Model file for the job. Use its own axes, mm. Coordinates: 2 decimals unless noted, no trailing zeros. Loops run counter-clockwise (first coordinate to the right, second up) from the corner with the lowest first, then second, coordinate; pieces in that order, holes last. Notation, with made-up numbers: (64.5, 7.5) -> (113.5, 7.5) arc R33 ccw to (113.5, 38.5) -> close; hole circle Ø9 at (78.5, -25). An arc over 180 degrees is marked (long way). Use one line per item in the form item = value.
```python
from build123d import *

# Parameters (mm, degrees)
F0_W     = 80
F0_H     = 80
F1_DEPTH = 3
F2_D     = 5.2
F3_R     = 10


with BuildPart() as f1:
    # F0 (on Top) → F1 (new body)
    with BuildSketch(Plane.XY):
        Rectangle(F0_W, F0_H)
    extrude(amount=F1_DEPTH)

    # F2 (through all)
    with Locations(Plane(origin=(0, 0, 0), x_dir=(1, 0, 0), z_dir=(0, 0, -1))):
        with Locations((-30, 30), (-10, 30), (10, 30), (30, 30), (30, 10), (10, 10), (-10, 10), (-30, 10), (-30, -10), (-10, -10), (10, -10), (30, -10), (30, -30), (10, -30), (-10, -30), (-30, -30)):
            Hole(F2_D / 2)

    # F3
    f3_edges = [f1.edges().sort_by_distance(p)[0] for p in [
        (40, 40, 1.5),
        (-40, 40, 1.5),
        (-40, -40, 1.5),
        (40, -40, 1.5),
    ]]
    fillet(f3_edges, radius=F3_R)


solid = f1.part
```
Q1. Band-saw the part on D-D, the plane x = -35. Write the cut outline in (y, z), and give its area (3 significant figures).
Result:
outline = (-38.66, 0) -> (38.66, 0) -> (38.66, 3) -> (-38.66, 3) -> close
area = 232 mm2
Q2. Band-saw the part on B-B, the plane z = 1.1. State how many separate pieces and enclosed holes the cut face has, and give its area (3 significant figures).
Result:
separate_pieces = 1
enclosed_holes = 16
area = 5,970 mm2
Q3. Pin check, flat tip, straight feed: pin 1 Ø1.5 at (x, z) = (-32, 2) entering from -Y. Stop position of the tip, or through.
Result:
pin_1 = -39.92
Q4. Wall check: line 1 along X through (y, z) = (-30, 1.6); line 2 along Y through (x, z) = (9, 2.85). Give the ranges that are in metal, low to high.
Result:
line_1 = -40 to -32.6, -27.4 to -12.6, -7.4 to 7.4, 12.6 to 27.4, 32.6 to 40
line_2 = -40 to -32.4, -27.6 to -12.4, -7.6 to 7.6, 12.4 to 27.6, 32.4 to 40
Q5. Mould opens along Y. For faces 1 (the face through (36.99, -37.15, 1.52)), 2 (the face through (32.063, -8.418, 1.521)), 3 (the face through (-37.15, 36.99, 1.52)), 4 (the face through (32.6, 29.9, 1.5)) say: released by +Y, released by -Y, zero draft, split by the parting line, or undercut.
Result:
face_1 = released by -Y
face_2 = undercut
face_3 = released by +Y
face_4 = undercut
Q6. Band-saw the part on A-A, the plane y = -10. Write the cut outline in (x, z).
Result:
outline = (-40, 0) -> (-32.6, 0) -> (-32.6, 3) -> (-40, 3) -> close; (-27.4, 0) -> (-12.6, 0) -> (-12.6, 3) -> (-27.4, 3) -> close; (-7.4, 0) -> (7.4, 0) -> (7.4, 3) -> (-7.4, 3) -> close; (12.6, 0) -> (27.4, 0) -> (27.4, 3) -> (12.6, 3) -> close; (32.6, 0) -> (40, 0) -> (40, 3) -> (32.6, 3) -> close
